from build123d import *
from build123d.topology import SkipClean

# Parameters (mm, degrees)
SKETCH1_W           = 136
SKETCH1_H           = 40
SKETCH1_W_2         = 2
BOSS_EXTRUDE1_DEPTH = 8
SKETCH1_3_W         = 2
SKETCH1_3_H         = 40
BOSS_EXTRUDE2_DEPTH = 9
SKETCH2_W           = 10.875
SKETCH2_H           = 9
BOSS_EXTRUDE3_DEPTH = 1
BOSS_EXTRUDE4_START = 1
SKETCH2_3_W         = 10.875
SKETCH2_3_H         = 9
SKETCH2_3_W_2       = 17.05
SKETCH2_3_H_2       = 0.6
BOSS_EXTRUDE4_DEPTH = 1
SKETCH1_4_W         = 2
SKETCH1_4_H         = 40
BOSS_EXTRUDE5_DEPTH = 30
SKETCH3_R           = 12.1
CUT_EXTRUDE1_DEPTH  = 132
FILLET1_R           = 5
FILLET2_START       = -31
FILLET2_DEPTH       = 40
BOSS_EXTRUDE6_START = -2
BOSS_EXTRUDE6_DEPTH = 134
FILLET3_R           = 0.5
FILLET5_R           = 1


with BuildPart() as part:
    # Sketch1 → Boss-Extrude1 (new body)
    with BuildSketch(Plane(origin=(0, 0, 0), x_dir=(1, 0, 0), z_dir=(0, 1, 0))):
        Rectangle(SKETCH1_W, SKETCH1_H)
        with Locations((69, 0)):
            Rectangle(SKETCH1_W_2, SKETCH1_H)
        with Locations((-69, 0)):
            Rectangle(SKETCH1_W_2, SKETCH1_H)
    extrude(amount=BOSS_EXTRUDE1_DEPTH)

    # Sketch1<3> → Boss-Extrude2 (add)
    with BuildSketch(Plane(origin=(0, 0, 0), x_dir=(1, 0, 0), z_dir=(0, 1, 0))):
        with Locations((69, 0)):
            Rectangle(SKETCH1_3_W, SKETCH1_3_H)
    extrude(amount=-BOSS_EXTRUDE2_DEPTH)

    # Sketch2 → Boss-Extrude3 (add)
    with BuildSketch(Plane.ZY.offset(-68)):
        with Locations((14.5625, -4.5)):
            Rectangle(SKETCH2_W, SKETCH2_H)
        with Locations((-14.5625, -4.5)):
            Rectangle(SKETCH2_W, SKETCH2_H)
    extrude(amount=BOSS_EXTRUDE3_DEPTH)

    # Sketch2<3> → Boss-Extrude4 (add)
    with BuildSketch(Plane.ZY.offset(-68).offset(BOSS_EXTRUDE4_START)):
        Polygon((9.125, -9), (9.125, 0), (8.525, 0), (8.525, -0.6), (8.525, -9), align=None)
        with Locations((14.5625, -4.5)):
            Rectangle(SKETCH2_3_W, SKETCH2_3_H)
        with Locations((0, -0.3)):
            Rectangle(SKETCH2_3_W_2, SKETCH2_3_H_2)
        Polygon((-8.525, -0.6), (-8.525, 0), (-9.125, 0), (-9.125, -9), (-8.525, -9), align=None)
        with Locations((-14.5625, -4.5)):
            Rectangle(SKETCH2_3_W, SKETCH2_3_H)
    extrude(amount=BOSS_EXTRUDE4_DEPTH)

    # Sketch1<4> → Boss-Extrude5 (add)
    with BuildSketch(Plane(origin=(0, 0, 0), x_dir=(1, 0, 0), z_dir=(0, 1, 0))):
        with Locations((-69, 0)):
            Rectangle(SKETCH1_4_W, SKETCH1_4_H)
    extrude(amount=-BOSS_EXTRUDE5_DEPTH)

    # Sketch3 → Cut-Extrude1 (cut)
    with BuildSketch(Plane.ZY.offset(-64)):
        with Locations((0, -6.5)):
            Circle(SKETCH3_R)
    extrude(amount=CUT_EXTRUDE1_DEPTH, mode=Mode.SUBTRACT)

    # Fillet1
    fillet1_edges = [part.edges().sort_by_distance(p)[0] for p in [
        (-1, 0, -20),
        (-1, 0, 20),
    ]]
    fillet(fillet1_edges, radius=FILLET1_R)

    # Fillet2: read off the stored shape, not the designer's step
    # Fillet2 outline → Fillet2 (cut)
    with BuildSketch(Plane(origin=(0, 0, 0), x_dir=(1, 0, 0), z_dir=(0, 1, 0)).offset(FILLET2_START)):
        with BuildLine():
            Line((-70, -20), (-68, -20))
            ThreePointArc((-68, -20), (-69.414213562, -19.414213562), (-70, -18))
            Line((-70, -18), (-70, -20))
        make_face()
        with BuildLine():
            ThreePointArc((70, -18), (69.414213562, -19.414213562), (68, -20))
            Line((68, -20), (70, -20))
            Line((70, -20), (70, -18))
        make_face()
        with BuildLine():
            Line((-70, 20), (-70, 18))
            ThreePointArc((-70, 18), (-69.414213562, 19.414213562), (-68, 20))
            Line((-68, 20), (-70, 20))
        make_face()
        with BuildLine():
            ThreePointArc((68, 20), (69.414213562, 19.414213562), (70, 18))
            Line((70, 18), (70, 20))
            Line((70, 20), (68, 20))
        make_face()
    extrude(amount=FILLET2_DEPTH, mode=Mode.SUBTRACT)

    # Sketch3<3> → Boss-Extrude6 (add)
    with SkipClean():  # the faces are left unmerged after this step: merging them gives an invalid solid
        with BuildSketch(Plane.ZY.offset(-64).offset(BOSS_EXTRUDE6_START)):
            with BuildLine():
                Line((-11.655363572, 0), (-11.655363572, -3.25))
                ThreePointArc((-11.655363572, -3.25), (-11.050752229, -1.571422601), (-10.205880658, 0))
                Line((-10.205880658, 0), (-11.655363572, 0))
            make_face()
            with BuildLine():
                ThreePointArc((10.205880658, 0), (11.050752229, -1.571422601), (11.655363572, -3.25))
                Line((11.655363572, -3.25), (11.655363572, 0))
                Line((11.655363572, 0), (10.205880658, 0))
            make_face()
        extrude(amount=BOSS_EXTRUDE6_DEPTH)

    # Fillet3
    fillet3_edges = [part.edges().sort_by_distance(p)[0] for p in [
        (-1, -3.25, -11.655363572),
        (-1, -3.25, 11.655363572),
    ]]
    fillet(fillet3_edges, radius=FILLET3_R)

    # Fillet5
    # the kernel refuses this fillet: 1 mm, written as the material it takes off along each edge
    with BuildSketch(Plane(origin=(64, 0, -12.705880658), x_dir=(1, 0, 0), z_dir=(0, 0, 1))) as fillet5_piece_1_section:
        with BuildLine():
            CenterArc((FILLET5_R, FILLET5_R), FILLET5_R, 180, 90)
            Line((0, FILLET5_R), (0, 0))
            Line((0, 0), (FILLET5_R, 0))
        make_face()
    fillet5_piece_1 = extrude(amount=25.411761315, mode=Mode.PRIVATE)
    fillet5_piece_1 = fillet5_piece_1 & Plane(origin=(64, -6.5, 0), x_dir=(0, 0.5371900826446553, 0.8434612113833264), z_dir=(1, 0, 0)) * Cylinder(12.1, 55, mode=Mode.PRIVATE)
    add(fillet5_piece_1, mode=Mode.SUBTRACT)


solid = part.part
Geometry check sheet. Reference: the model listing, model coordinates, mm. A direction names the side the tool comes from. Give positions to 0.01 mm unless a question says otherwise; leave off trailing zeros. Order: outer loops, then holes, each group sorted by start corner. A loop starts at its lowest first (then second) coordinate and runs counter-clockwise, first axis right, second up.
1. Access from +Z, -Z, +X, -X, +Y, -Y to the whole of each face (thin tool, end or side, straight path). Record for faces 1 (the face through (-2, 0, 13)), 2 (the face through (-2, 0, -13)), 3 (the face through (-68, -12, 0)).
Completed:
face 1: +Z, -Y
face 2: -Z, -Y
face 3: -Y
2. Depth check by flat-ended pin: pin 1 (0.5 mm diameter, centred on x = -22, y = -0.5, fed in from +Z); pin 2 (0.8 mm diameter, centred on x = 67.5, z = -4, fed in from -Y); pin 3 (10 mm diameter, centred on x = -44.5, z = 9.5, fed in from -Y). Enter the tip coordinate at first touch or a pass-through.
Completed:
pin 1: stops at z = 11.66
pin 2: stops at y = 0
pin 3: stops at y = -1.14
3. Sectioned sample at A-A (y = -4). Record the boundary of the cut face in (x, z) (3 decimals).
Completed:
outline: (-70, -18) arc R2 ccw to (-68, -20) - (-68, 20) arc R2 ccw to (-70, 18) - close; (66, -20) - (68, -20) arc R2 ccw to (70, -18) - (70, 18) arc R2 ccw to (68, 20) - (66, 20) - (66, 8.525) - (67, 8.525) - (67, 9.125) - (68, 9.125) - (68, -9.125) - (67, -9.125) - (67, -8.525) - (66, -8.525) - close
4. Scan lines: line 1 (X direction, y = 1.5, z = 5); line 2 (X direction, y = -4.5, z = 12.5); line 3 (Y direction, x = 8.5, z = 0). Record each from-to range of solid material in increasing order.
Completed:
line 1: x = -70 to -68, 64 to 70
line 2: x = -70 to -68, 66 to 70
line 3: y = 5.6 to 8
5. Sectioned sample at B-B (x = -20.5). Record the boundary of the cut face in (y, z).
Completed:
outline: (-0.87, -10.71) arc R0.5 ccw to (-0.64, -11.66) - (0, -11.66) - (0, -15) arc R5 ccw to (5, -20) - (8, -20) - (8, 20) - (5, 20) arc R5 ccw to (0, 15) - (0, 11.66) - (-0.64, 11.66) arc R0.5 ccw to (-0.87, 10.71) arc R12.1 cw to start
6. Draft check along X on faces 4 (the face through (70, 0, 0)), 5 (the face through (68, -4, 0)), 6 (the face through (-70, -11, 0)), 7 (the face through (68.5, -9, -0.3)). Enter one of: pulls with the +X half, pulls with the -X half, needs draft (parallel to the pull), parting line crosses it, or undercut.
Completed:
face 4: pulls with the +X half
face 5: undercut
face 6: pulls with the -X half
face 7: needs draft
7. Sectioned sample at D-D (y = -23.5). Record the boundary of the cut face in (x, z).
Completed:
outline: (-70, -18) arc R2 ccw to (-68, -20) - (-68, 20) arc R2 ccw to (-70, 18) - close
8. Sectioned sample at C-C (z = 16.5). Record the boundary of the cut face in (x, y).
Completed:
outline: (-70, -30) - (-68, -30) - (-68, 0.23) - (66, 0.23) - (66, -9) - (70, -9) - (70, 8) - (-70, 8) - close
